```python
from build123d import *

# Parameters (mm, degrees)
F0_R     = 38
F1_DEPTH = 30
F2_R     = 35
F2_R_2   = 17.5
F3_DEPTH = 27
F5_START = 11
F4_R     = 12.8
F5_DEPTH = 35
F7_DEPTH = 27
F8_R     = 1.55
F9_DEPTH = 5


with BuildPart() as f1:
    # F0 (on Top) → F1 (new body)
    with BuildSketch(Plane.XY):
        Circle(F0_R)
    extrude(amount=F1_DEPTH)

    # F2 (on face) → F3 (cut)
    with BuildSketch(Plane(origin=(0, 0, 0), x_dir=(1, 0, 0), z_dir=(0, 0, -1))):
        Circle(F2_R)
        Circle(F2_R_2, mode=Mode.SUBTRACT)
    extrude(amount=-F3_DEPTH, mode=Mode.SUBTRACT)

    # F4 (on Right) → F5 (cut)
    with BuildSketch(Plane.YZ.offset(F5_START)):
        with Locations((0, 15)):
            Circle(F4_R)
    extrude(amount=F5_DEPTH, mode=Mode.SUBTRACT)

    # F6 (on face) → F7 (cut)
    with BuildSketch(Plane(origin=(0, 0, 0), x_dir=(1, 0, 0), z_dir=(0, 0, -1))):
        with BuildLine():
            Line((8, -10.8742815855), (8, 10.8742815855))
            ThreePointArc((8, 10.8742815855), (-13.5, 0), (8, -10.8742815855))
        make_face()
    extrude(amount=-F7_DEPTH, mode=Mode.SUBTRACT)

    # F8 (on face) → F9 (cut)
    with BuildSketch(Plane.YZ.offset(11)):
        with Locations((0, 15)):
            Circle(F8_R)
    extrude(amount=-F9_DEPTH, mode=Mode.SUBTRACT)


solid = f1.part
```
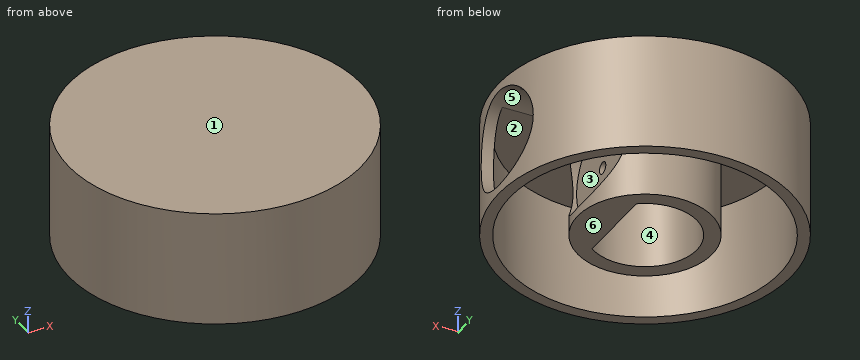
Geometry check sheet. Reference: the model listing, model coordinates, mm. Face numbers are marked on the shaded views. A direction names the side the tool comes from. Give positions to 0.01 mm unless a question says otherwise; leave off trailing zeros. Write each loop counter-clockwise with the first axis right and the second up, starting at its lowest first coordinate (ties: lowest second). Pieces come first, ordered by that corner, then holes.
1) Release check for a two-part mould opening along Z. For the marked faces 4, 5 and 6 record: pulls with the +Z half, pulls with the -Z half, needs draft (parallel to the pull), parting line crosses it, or undercut.
2) Section check D-D, the plane z = 15. Record the boundary of the cut face in (x, y).
3) Access from +Z, -Z, +X, -X, +Y, -Y to the whole of each face (thin tool, end or side, straight path). Record for the marked faces 1, 2 and 3.
4) Section check A-A, the plane z = 20.5. Record the boundary of the cut face in (x, y), and give its area (3 significant figures).
5) Section check C-C, the plane x = 15.5. Record the boundary of the cut face in (y, z), and give its area (3 significant figures).
6) Material ranges on L1, parallel to Y at x = 0, z = 10.5; L2, parallel to X at y = -11, z = 26; L3, parallel to Z at x = 4, y = 23, recorded low to high.
7) Section check B-B, the plane y = 0. Record the boundary of the cut face in (x, z), and give its area (3 significant figures).
8) Gauge pin test, flat ends, axial feed: pin 1 (4 mm diameter, centred on x = -4, y = -30, fed in from -Z); pin 2 (3 mm diameter, centred on y = -26, z = 11.5, fed in from -X); pin 3 (5 mm diameter, centred on x = -11, z = 17.5, fed in from -Y). Record the tip position at first contact, or that the pin passes through.
Computed:
1. face 4: needs draft
1. face 5: undercut
1. face 6: pulls with the -Z half
2. outline: (8, -10.87) arc R13.5 cw (long way) to (8, 10.87) - (8, 1.55) - (11, 1.55) - (11, 12.8) - (11.93, 12.8) arc R17.5 ccw (long way) to (11.93, -12.8) - (11, -12.8) - (11, -1.55) - (8, -1.55) - close; (32.58, -12.8) arc R35 cw (long way) to (32.58, 12.8) - (35.78, 12.8) arc R38 ccw (long way) to (35.78, -12.8) - close
3. face 1: +Z, +X, -X, +Y, -Y
3. face 2: -Z
3. face 3: +X
4. outline: (11, -11.56) - (11, 11.56) - (13.14, 11.56) arc R17.5 ccw (long way) to (13.14, -11.56) - close; (33.04, -11.56) arc R35 cw (long way) to (33.04, 11.56) - (36.2, 11.56) arc R38 ccw (long way) to (36.2, -11.56) - close; hole (8, -10.87) - (8, 10.87) arc R13.5 ccw (long way) to start
4. area: 972 mm2
5. outline: (-34.7, 0) - (-31.38, 0) - (-31.38, 27) - (-8.12, 27) - (-8.12, 24.89) arc R12.8 cw to (8.12, 24.89) - (8.12, 27) - (31.38, 27) - (31.38, 0) - (34.7, 0) - (34.7, 30) - (-34.7, 30) - close; (-8.12, 0) - (8.12, 0) - (8.12, 5.11) arc R12.8 cw to (-8.12, 5.11) - close
5. area: 440 mm2
6. L1: y = -38 to -35, -17.5 to -13.5, 13.5 to 17.5, 35 to 38
6. L2: x = -36.37 to -33.23, -13.61 to -7.83, 7.83 to 13.61, 33.23 to 36.37
6. L3: z = 27 to 30
7. outline: (-38, 0) - (-35, 0) - (-35, 27) - (-17.5, 27) - (-17.5, 0) - (-13.5, 0) - (-13.5, 27) - (8, 27) - (8, 16.55) - (11, 16.55) - (11, 27.8) - (38, 27.8) - (38, 30) - (-38, 30) - close; (8, 0) - (17.5, 0) - (17.5, 2.2) - (11, 2.2) - (11, 13.45) - (8, 13.45) - close; (35, 0) - (38, 0) - (38, 2.2) - (35, 2.2) - close
7. area: 488 mm2
8. pin 1: stops at z = 27
8. pin 2: stops at x = -29.05
8. pin 3: stops at y = -37.04
